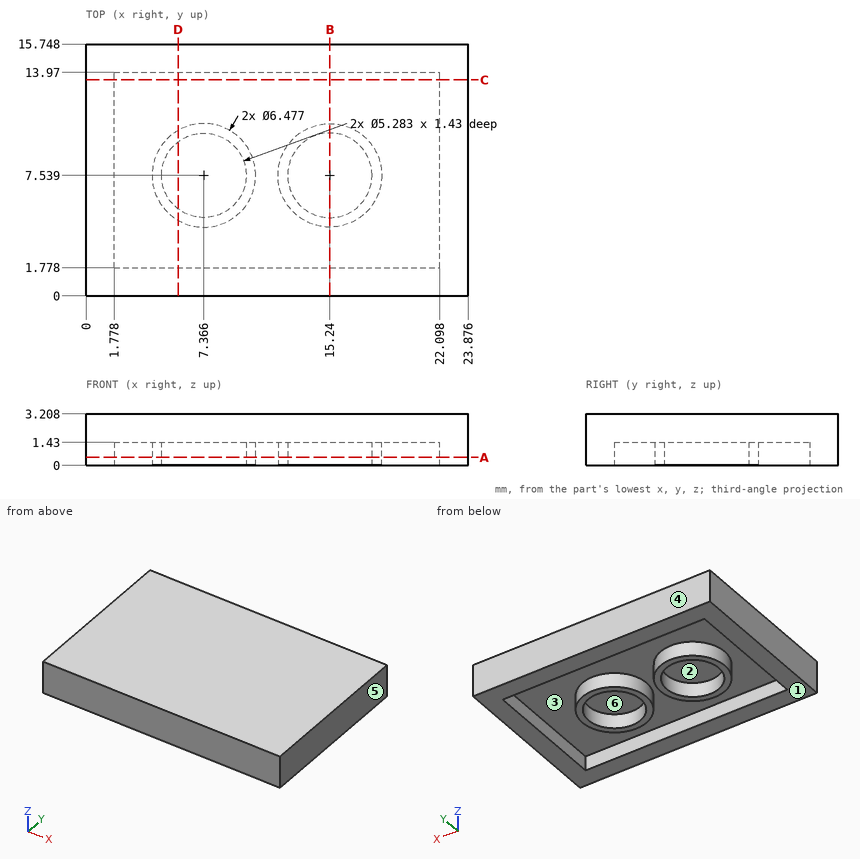
Here's the drawing with two shaded views (mm, measured from the low corner). I have some questions. A direction names the side the tool comes from. Coordinates: 2 decimals unless noted, no trailing zeros. Order: outer loops, then holes, each group sorted by start corner. A loop starts at its lowest first (then second) coordinate and runs counter-clockwise, first axis right, second up. Notation, with made-up numbers: (46, 82) - (96, 82) arc R8 cw to (96, 94) - close; hole circle Ø1 at (52.25, 88.25). An arc over 180 degrees is marked (long way). Use CSV: the item, a comma, the result in double quotes. Start each with the question number.
1. Please list where these lines run through material, in increasing order: line 1 (Y direction, x = 7.5, z = 0.3) (1 decimal); line 2 (Y direction, x = 22, z = 0.65); line 3 (X direction, y = 2.25, z = 0.4). Write a range as from..to.
2. For the marked faces 5 and 6, which set-ups out of +Z, -Z, +X, -X, +Y, -Y let a thin tool reach every point of the face, with its end or its side?
3. I'm going to push a flat-ended pin straight in: pin 1 (1.6 mm diameter, centred on x = 7, y = 8.5, fed in from -Z). Where does the tip first touch, or does it pass through?
4. If we mould it in two halves opening along Y, with no side actions, what happens to the marked faces 1, 2, 3 and 4? For each: +Y half, -Y half, draft (parallel to the pull), parting line (faces both ways), or undercut.
5. Suppose I cut it at B-B on x = 15.24. List the corners of the cut face in (y, z) for me.
6. Suppose I cut it at A-A on z = 0.5. List the corners of the cut face in (x, y) for me.
7. Suppose I cut it at C-C on y = 13.5. List the corners of the cut face in (x, z) for me.
8. Suppose I cut it at D-D on x = 5.75. List the corners of the cut face in (y, z) for me (1 decimal).
Output:
1,line 1,"y = 0..1.8, 4.3..4.9, 10.2..10.8, 14..15.7"
1,line 2,"y = 0..1.78, 13.97..15.75"
1,line 3,"x = 0..1.78, 22.1..23.88"
2,face 5,"+Z, -Z, +X, +Y, -Y"
2,face 6,"-Z"
3,pin 1,"stops at z = 1.43"
4,face 1,"draft"
4,face 2,"undercut"
4,face 3,"undercut"
4,face 4,"+Y half"
5,outline,"(0, 0) - (1.78, 0) - (1.78, 1.43) - (4.3, 1.43) - (4.3, 0) - (4.9, 0) - (4.9, 1.43) - (10.18, 1.43) - (10.18, 0) - (10.78, 0) - (10.78, 1.43) - (13.97, 1.43) - (13.97, 0) - (15.75, 0) - (15.75, 3.21) - (0, 3.21) - close"
6,outline,"(0, 0) - (23.88, 0) - (23.88, 15.75) - (0, 15.75) - close; circle Ø6.48 at (7.37, 7.54); circle Ø6.48 at (15.24, 7.54); hole (1.78, 1.78) - (22.1, 1.78) - (22.1, 13.97) - (1.78, 13.97) - close; hole circle Ø5.28 at (7.37, 7.54); hole circle Ø5.28 at (15.24, 7.54)"
7,outline,"(0, 0) - (1.78, 0) - (1.78, 1.43) - (22.1, 1.43) - (22.1, 0) - (23.88, 0) - (23.88, 3.21) - (0, 3.21) - close"
8,outline,"(0, 0) - (1.8, 0) - (1.8, 1.4) - (4.7, 1.4) - (4.7, 0) - (5.4, 0) - (5.4, 1.4) - (9.6, 1.4) - (9.6, 0) - (10.3, 0) - (10.3, 1.4) - (14, 1.4) - (14, 0) - (15.7, 0) - (15.7, 3.2) - (0, 3.2) - close"
